Source: CAD feature listing. Evaluate the final solid. Frame: model axes, mm. Coordinates: 2 decimals unless noted, no trailing zeros. Order: outer loops, then holes, each group sorted by start corner. A loop starts at its lowest first (then second) coordinate and runs counter-clockwise, first axis right, second up.
Autodesk Inventor part; units mm, degrees
ref_plane "YZ Plane" through (0, 0, 0) normal (1, 0, 0) x (0, 1, 0)
ref_plane "XZ Plane" through (0, 0, 0) normal (0, 1, 0) x (-1, 0, 0)
ref_plane "XY Plane" through (0, 0, 0) normal (0, 0, 1) x (1, 0, 0)
sketch "スケッチ1" plane through (0, 0, 0) normal (0, 1, 0) x (-1, 0, 0)
  circle A0 centre (0, 0) radius 8.25 construction
  circle A1 centre (0, 0) radius 12
  circle A2 centre (0, 0) radius 10.125 construction
  circle A3 centre (10.125, 0) radius 1
  line L0 (16.8, 0) -> (-16.8, 0)
  circle A4 centre (5.0625, 8.7685) radius 1
  circle A5 centre (-5.0625, 8.7685) radius 1
  circle A6 centre (-10.125, 0) radius 1
  circle A7 centre (-5.0625, -8.7685) radius 1
  circle A8 centre (5.0625, -8.7685) radius 1
  circle A9 centre (0, 0) radius 4.25
  dimension "d3" = 20.25
  dimension "d0" = 16.5
  dimension "d1" = 24
  dimension "d4" = 2
  dimension "d7" = 360
  dimension "d9" = 8.5
extrude "プレート1" add sketch "スケッチ1" along normal blind 1.5 contours L0 A3 A9 A6 A1 | A1 L0 A6 A9 A3
sketch "スケッチ2" plane through (0, 0, 0) normal (0, -1, 0) x (1, 0, 0)
  circle A0 centre (5.1962, -3) radius 1
  circle A1 centre (5.7956, 1.5529) radius 1
  circle A2 centre (3, 5.1962) radius 1
  circle A3 centre (-5.7956, -1.5529) radius 1
  line L0 (17.8564, -1.0718) -> (9.8564, -14.9282)
  line L1 (-17.8564, 1.0718) -> (-12.4853, -2.0292)
  arc A4 (11.5588, 3.2239) -> (-2.9874, 11.6222) centre (0, 0) ccw
  line L2 (4.4853, -11.8272) -> (9.8564, -14.9282)
  line L3 (-17.8564, 1.0718) -> (-9.8564, 14.9282)
  line L4 (17.8564, -1.0718) -> (12.4853, 2.0292)
  arc A5 (-11.5588, -3.2239) -> (2.9874, -11.6222) centre (0, 0) ccw
  line L5 (-4.4853, 11.8272) -> (-9.8564, 14.9282)
  circle A6 centre (-5.7956, -1.5529) radius 1
  circle A7 centre (-3, -5.1962) radius 1
  circle A8 centre (0, 0) radius 4.25
  circle A9 centre (1.5529, -5.7956) radius 1
  circle A10 centre (5.1962, -3) radius 1
  circle A11 centre (5.7956, 1.5529) radius 1
  circle A12 centre (3, 5.1962) radius 1
  circle A13 centre (1.5529, -5.7956) radius 1
  circle A14 centre (-5.0625, 8.7685) radius 1
  circle A15 centre (-5.0625, -8.7685) radius 1
  circle A16 centre (10.125, 0) radius 1
  circle A17 centre (5.0625, -8.7685) radius 1
  circle A18 centre (-10.125, 0) radius 1
  circle A19 centre (5.0625, 8.7685) radius 1
  arc A20 (4.4853, -11.8272) -> (2.9874, -11.6222) centre (3.4853, -13.5592) ccw
  arc A21 (-11.5588, -3.2239) -> (-12.4853, -2.0292) centre (-13.4853, -3.7613) ccw
  arc A22 (-4.4853, 11.8272) -> (-2.9874, 11.6222) centre (-3.4853, 13.5592) ccw
  arc A23 (11.5588, 3.2239) -> (12.4853, 2.0292) centre (13.4853, 3.7613) ccw
  circle A24 centre (-5.1962, 3) radius 1
  circle A25 centre (-1.5529, 5.7956) radius 1
  point P0 (0, 0)
  point P1 (0, 0)
  point P2 (0, 0)
  point P3 (0, 0)
  point P4 (0, 0)
  point P5 (9.798, -10)
  point P6 (-9.798, -10)
  point P7 (-9.798, 10)
  point P8 (9.798, 10)
extrude "切り取り1" cut sketch "スケッチ2" against normal blind 1.5 contours A0 | A1 | A2 | A3 | A7 | A9 | A24 | A25
equation "\"d3\" = 0.5 * d0 + 0.5 * d1"
equation "\"d10\" = Thickness"
equation "\"d2\" = Thickness"
equation "\"BendRadius\" = Thickness"
equation "\"BendReliefWidth\" = Thickness"
equation "\"BendReliefDepth\" = 0.5 * Thickness"
equation "\"CornerReliefSize\" = 4 * Thickness"
equation "\"MinimumRemnant\" = 2 * Thickness"
equation "\"TransitionRadius\" = BendRadius"
equation "\"JacobiRadiusSize\" = BendRadius"
equation "\"GapSize\" = Thickness"
properties part number "sholder_joint_s" material "アルミニウム 6061"
1. Section query B-B on z = -3. Return loops of the section in (x, y), plus the area to 3 significant figures.
Findings:
outline: (-11.62, 0) - (-3.01, 0) - (-3.01, 1.5) - (-11.62, 1.5) - close; (3.01, 0) - (4.2, 0) - (4.2, 1.5) - (3.01, 1.5) - close; (6.2, 0) - (11.62, 0) - (11.62, 1.5) - (6.2, 1.5) - close
area: 22.8 mm2
2. Section query D-D on y = 0.3. Count the separate pieces of the cut face and the enclosed holes in it, plus the area to 3 significant figures.
Findings:
separate pieces: 1
enclosed holes: 15
area: 352 mm2
3. Section query A-A on z = 0. Return loops of the section in (x, y) (3 decimals), plus the area to 4 significant figures.
Findings:
outline: (-12, 0) - (-11.125, 0) - (-11.125, 1.5) - (-12, 1.5) - close; (-9.125, 0) - (-4.25, 0) - (-4.25, 1.5) - (-9.125, 1.5) - close; (4.25, 0) - (9.125, 0) - (9.125, 1.5) - (4.25, 1.5) - close; (11.125, 0) - (12, 0) - (12, 1.5) - (11.125, 1.5) - close
area: 17.25 mm2
4. Ray query, line 1 (X direction, y = 0.75, z = 0) (3 decimals); line 2 (Z direction, x = -1, y = 1); line 3 (Z direction, x = -5, y = 0.15). Return the intervals inside material, ascending.
Findings:
line 1: x = -12 to -11.125, -9.125 to -4.25, 4.25 to 9.125, 11.125 to 12
line 2: z = -11.96 to -4.13, 4.13 to 4.96, 6.63 to 11.96
line 3: z = -10.91 to -9.77, -7.77 to -2.16, -0.95 to 2.02, 3.98 to 7.77, 9.77 to 10.91
5. Pin query (flat end, axial travel): P1, Ø2.5, axis at x = -3, z = -5.2, coming from the -Y side. Return the tip coordinate at first contact, or that it passes through.
Findings:
P1: stops at y = 0
6. Section query C-C on x = 3. Return loops of the section in (y, z), plus the area to 3 significant figures.
Findings:
outline: (0, -11.62) - (1.5, -11.62) - (1.5, -3.01) - (0, -3.01) - close; (0, 3.01) - (1.5, 3.01) - (1.5, 4.2) - (0, 4.2) - close; (0, 6.2) - (1.5, 6.2) - (1.5, 11.62) - (0, 11.62) - close
area: 22.8 mm2
7. Draft query along X for faces 1 (the face through (11.99, 0.74, -0.53)), 2 (the face through (0, 0, -5)), 3 (the face through (6.75, 0.74, 1.85)). Return one class per face: released by +X, released by -X, zero draft, split by the parting line, or undercut.
Findings:
face 1: split by the parting line
face 2: zero draft
face 3: undercut
